from build123d import *

# Parameters (mm, degrees)
F0_R     = 11
F0_R_2   = 10.925
F1_DEPTH = 7
F2_R     = 4
F3_SIZE  = 1
F4_R     = 11.925
F4_R_2   = 11.25
F4_R_3   = 12
F5_DEPTH = 7


# Not quite as in the source:
# - a feature names something its author has since deleted; it is built from what else it names


with BuildPart() as f1:
    # F0 (on Top) → F1 (new body)
    with BuildSketch(Plane.XY):
        with BuildLine():
            Line((20.8717118949, 34.490134567), (0, 45))
            Line((0, 45), (-20.8717118949, 34.490134567))
            Line((-20.8717118949, 34.490134567), (-9.8614735953, 11.3027137683))
            ThreePointArc((-9.8614735953, 11.3027137683), (0, 15), (9.8614735953, 11.3027137683))
            Line((9.8614735953, 11.3027137683), (20.8717118949, 34.490134567))
        make_face()
        with Locations((0, 27.5248214602)):
            Circle(F0_R, mode=Mode.SUBTRACT)
        with BuildLine():
            ThreePointArc((9.8614735953, 11.3027137683), (0, 15), (-9.8614735953, 11.3027137683))
            ThreePointArc((-9.8614735953, 11.3027137683), (-12.9903810568, 7.5), (-14.7191740527, 2.8889297681))
            ThreePointArc((-14.7191740527, 2.8889297681), (-12.9903810568, -7.5), (-4.8577004574, -14.1916435365))
            ThreePointArc((-4.8577004574, -14.1916435365), (0, -15), (4.8577004574, -14.1916435365))
            ThreePointArc((4.8577004574, -14.1916435365), (12.2038007781, -8.7216538896), (15, 0))
            ThreePointArc((15, 0), (14.9296284413, 1.4512734423), (14.7191740527, 2.8889297681))
            ThreePointArc((14.7191740527, 2.8889297681), (12.9903810568, 7.5), (9.8614735953, 11.3027137683))
        make_face()
        Circle(F0_R_2, mode=Mode.SUBTRACT)
        with BuildLine():
            ThreePointArc((-4.8577004574, -14.1916435365), (-12.9903810568, -7.5), (-14.7191740527, 2.8889297681))
            Line((-14.7191740527, 2.8889297681), (-40.3051886624, 0.8303654379))
            Line((-40.3051886624, 0.8303654379), (-38.9711431703, -22.5))
            Line((-38.9711431703, -22.5), (-19.4334767676, -35.3205000049))
            Line((-19.4334767676, -35.3205000049), (-4.8577004574, -14.1916435365))
        make_face()
        with Locations((-23.8371946192, -13.7624107301)):
            Circle(F0_R, mode=Mode.SUBTRACT)
        with BuildLine():
            Line((40.3051886624, 0.8303654379), (14.7191740527, 2.8889297681))
            ThreePointArc((14.7191740527, 2.8889297681), (14.9296284413, 1.4512734423), (15, 0))
            ThreePointArc((15, 0), (12.2038007781, -8.7216538896), (4.8577004574, -14.1916435365))
            Line((4.8577004574, -14.1916435365), (19.4334767676, -35.3205000049))
            Line((19.4334767676, -35.3205000049), (38.9711431703, -22.5))
            Line((38.9711431703, -22.5), (40.3051886624, 0.8303654379))
        make_face()
        with Locations((23.8371946192, -13.7624107301)):
            Circle(F0_R, mode=Mode.SUBTRACT)
    extrude(amount=F1_DEPTH)

    # F2
    f2_edges = [f1.edges().sort_by_distance(p)[0] for p in [
        (9.861474, 11.302714, 3.5),
        (-9.861474, 11.302714, 3.5),
        (14.719174, 2.88893, 3.5),
        (4.8577, -14.191644, 3.5),
        (-4.8577, -14.191644, 3.5),
        (-14.719174, 2.88893, 3.5),
        (20.871712, 34.490135, 3.5),
        (0, 45, 3.5),
        (-20.871712, 34.490135, 3.5),
        (19.433477, -35.3205, 3.5),
        (38.971143, -22.5, 3.5),
        (40.305189, 0.830365, 3.5),
        (-19.433477, -35.3205, 3.5),
        (-38.971143, -22.5, 3.5),
        (-40.305189, 0.830365, 3.5),
    ]]
    fillet(f2_edges, radius=F2_R)

    # F3
    f3_edges = [f1.edges().sort_by_distance(p)[0] for p in [
        (-15.121499, 22.38026, 7),
        (-15.121499, 22.38026, 0),
        (-39.584098, -11.780379, 7),
        (-29.994156, -28.390645, 7),
        (15.121499, 22.38026, 7),
        (10.691316, 11.594325, 7),
        (19.36544, 33.973357, 7),
        (12.990381, 7.5, 7),
        (9.589942, 40.171024, 7),
        (15.386638, 3.461789, 7),
        (0, 44.521503, 7),
        (26.942623, 1.905472, 7),
        (-9.589942, 40.171024, 7),
        (39.10451, -0.215715, 7),
        (-19.36544, 33.973357, 7),
        (39.584098, -11.780379, 7),
        (38.556753, -22.260751, 7),
        (-10.691316, 11.594325, 7),
        (29.994156, -28.390645, 7),
        (-12.990381, 7.5, 7),
        (19.73907, -33.757641, 7),
        (-15.386638, 3.461789, 7),
        (11.821124, -24.285733, 7),
        (-26.942623, 1.905472, 7),
        (4.695322, -15.056114, 7),
        (-39.10451, -0.215715, 7),
        (0, -15, 7),
        (-4.695322, -15.056114, 7),
        (-38.556753, -22.260751, 7),
        (-11.821124, -24.285733, 7),
        (-19.73907, -33.757641, 7),
        (-11, 27.524821, 7),
        (-10.925, 0, 7),
        (-34.837195, -13.762411, 7),
        (12.837195, -13.762411, 7),
        (15.121499, 22.38026, 0),
        (10.691316, 11.594325, 0),
        (19.36544, 33.973357, 0),
        (12.990381, 7.5, 0),
        (9.589942, 40.171024, 0),
        (15.386638, 3.461789, 0),
        (0, 44.521503, 0),
        (26.942623, 1.905472, 0),
        (-9.589942, 40.171024, 0),
        (39.10451, -0.215715, 0),
        (-19.36544, 33.973357, 0),
        (39.584098, -11.780379, 0),
        (38.556753, -22.260751, 0),
        (-10.691316, 11.594325, 0),
        (29.994156, -28.390645, 0),
        (-12.990381, 7.5, 0),
        (19.73907, -33.757641, 0),
        (-15.386638, 3.461789, 0),
        (11.821124, -24.285733, 0),
        (-26.942623, 1.905472, 0),
        (4.695322, -15.056114, 0),
        (-39.10451, -0.215715, 0),
        (0, -15, 0),
        (-39.584098, -11.780379, 0),
        (-4.695322, -15.056114, 0),
        (-38.556753, -22.260751, 0),
        (-11.821124, -24.285733, 0),
        (-29.994156, -28.390645, 0),
        (-19.73907, -33.757641, 0),
        (-11, 27.524821, 0),
        (-10.925, 0, 0),
        (-34.837195, -13.762411, 0),
        (12.837195, -13.762411, 0),
    ]]
    chamfer(f3_edges, length=F3_SIZE)

    # F4 (on face) → F5 (join)
    with BuildSketch(Plane.XY.offset(7)):
        Circle(F4_R)
        Circle(F4_R_2, mode=Mode.SUBTRACT)
        with Locations((0, 27.5248214602)):
            Circle(F4_R_3)
        with Locations((0, 27.5248214602)):
            Circle(F4_R_2, mode=Mode.SUBTRACT)
        with Locations((-23.8371946192, -13.7624107301)):
            Circle(F4_R_3)
        with Locations((-23.8371946192, -13.7624107301)):
            Circle(F4_R_2, mode=Mode.SUBTRACT)
        with Locations((23.8371946192, -13.7624107301)):
            Circle(F4_R_3)
        with Locations((23.8371946192, -13.7624107301)):
            Circle(F4_R_2, mode=Mode.SUBTRACT)
    extrude(amount=-F5_DEPTH)


solid = f1.part
Read the model definition and answer for the solid it produces. Units are mm, in the model's axes. A direction names the side the tool comes from. Give positions to 0.01 mm unless a question says otherwise; leave off trailing zeros. Write each loop counter-clockwise with the first axis right and the second up, starting at its lowest first coordinate (ties: lowest second). Pieces come first, ordered by that corner, then holes. Notation, with made-up numbers: M 72.5,83.5 L 100.5,83.5 A9 cw 100.5,91.5 Z; hole C -12.5,33 d11. An arc over 180 degrees is marked long. One line per item, written item: value. Start each with the question number.
(1) Find section A-A (x = 0). Give the number of separate pieces and of enclosed holes in the cut face, plus the area to 3 significant figures.
(2) Find the intervals of material crossed by line 1 (X direction, y = -14, z = 4.5); line 2 (Y direction, x = 1, z = 1.5); line 3 (X direction, y = -23, z = 4.75), in increasing order.
(3) A tool of negligible diameter and unlimited length cuts with its end or side. For faces 4 (the cylindrical face through (-15.36, 3.48, 3.54)), 5 (the flat face through (12.15, -23.9, 6.49)), 6 (the flat face through (15.064, 22.26, 3.465)), 7 (the flat face through (-11.9, -24.4, 3.5)), 8 (the cylindrical face through (12.598, -13.268, 0.38)), from which of +Z, -Z, +X, -X, +Y, -Y can it reach the whole face along a straight path? Write none if from no direction.
(4) Determine the mould class of faces 1 (the flat face through (9.48, 39.68, 6.49)), 2 (the conical face through (-19.91, -33.06, 0.28)), 3 (the conical face through (18.7, 33.708, 6.715)) for opening direction Y: pulls with the +Y half, pulls with the -Y half, needs draft (parallel to the pull), parting line crosses it, or undercut.
(5) Flat-ended cylindrical pins translate along their axes: pin 1 Ø1 at (y, z) = (8.5, 3) entering from +X; pin 2 Ø2 at (y, z) = (-17.5, 4) entering from +X; pin 3 Ø20 at (x, y) = (23.84, -13.76) entering from +Z; pin 4 Ø4 at (x, z) = (-11.5, 2.5) entering from -Y. Find the tip coordinate at first contact, or state that the pin passes through.
(6) Find section C-C (y = -26). Determine the outline of the cut face in (x, z), plus the area to 3 significant figures.
Results below:
1. separate pieces: 3
1. enclosed holes: 0
1. area: 106 mm^2
2. line 1: x = -39.46 to -34.83, -12.84 to 12.84, 34.83 to 39.46
2. line 2: y = -14.97 to -10.88, 10.88 to 16.57, 38.48 to 44.39
2. line 3: x = -38.01 to -29.81, -17.87 to -10.93, 10.93 to 17.87, 29.81 to 38.01
3. face 4: +Z, -Z, -X
3. face 5: +Z, -Y
3. face 6: +Z, -Z, +X
3. face 7: +Z, -Z, -Y
3. face 8: -Z
4. face 1: pulls with the +Y half
4. face 2: pulls with the -Y half
4. face 3: undercut
5. pin 1: stops at x = 12.69
5. pin 2: stops at x = 39.31
5. pin 3: passes through
5. pin 4: stops at y = -26.72
6. outline: M -33.64,1 L -31.81,0 L -14.22,0 L -13,1 L -13,6 L -14.22,7 L -31.81,7 L -33.64,6 Z; M 13,1 L 14.22,0 L 31.81,0 L 33.64,1 L 33.64,6 L 31.81,7 L 14.22,7 L 13,6 Z
6. area: 283 mm^2
